```python
from build123d import *

# Parameters (mm, degrees)
F1_DEPTH = 2.7
F3_DEPTH = 6.2
F4_R     = 1.25
F5_DEPTH = 25
F6_SIZE  = 0.5


with BuildPart() as f1:
    # F0 (on Top) → F1 (new body)
    with BuildSketch(Plane.XY):
        with BuildLine():
            Line((-35, -6), (35, -6))
            ThreePointArc((35, -6), (36.3416407865, -5.683281573), (37.4, -4.8))
            ThreePointArc((37.4, -4.8), (39, 0), (37.4, 4.8))
            ThreePointArc((37.4, 4.8), (36.3416407865, 5.683281573), (35, 6))
            Line((35, 6), (-35, 6))
            ThreePointArc((-35, 6), (-36.3416407865, 5.683281573), (-37.4, 4.8))
            ThreePointArc((-37.4, 4.8), (-39, 0), (-37.4, -4.8))
            ThreePointArc((-37.4, -4.8), (-36.3416407865, -5.683281573), (-35, -6))
        make_face()
    extrude(amount=F1_DEPTH)

    # F2 (on face) → F3 (join)
    with BuildSketch(Plane.XY.offset(2.7)):
        with BuildLine():
            Line((29, 4.5), (-29, 4.5))
            ThreePointArc((-29, 4.5), (-31.8284271247, 3.3284271247), (-33, 0.5))
            Line((-33, 0.5), (-33, -0.5))
            ThreePointArc((-33, -0.5), (-31.8284271247, -3.3284271247), (-29, -4.5))
            Line((-29, -4.5), (29, -4.5))
            ThreePointArc((29, -4.5), (31.8284271247, -3.3284271247), (33, -0.5))
            Line((33, -0.5), (33, 0.5))
            ThreePointArc((33, 0.5), (31.8284271247, 3.3284271247), (29, 4.5))
        make_face()
    extrude(amount=F3_DEPTH)

    # F4 (on face) → F5 (cut)
    with BuildSketch(Plane.XY.offset(2.7)):
        with Locations((-36.5, 0)):
            Circle(F4_R)
        with Locations((36.5, 0)):
            Circle(F4_R)
    extrude(amount=-F5_DEPTH, mode=Mode.SUBTRACT)

    # F6
    f6_edges = [f1.edges().sort_by_distance(p)[0] for p in [
        (-37.75, 0, 0),
        (35.25, 0, 0),
    ]]
    chamfer(f6_edges, length=F6_SIZE)


solid = f1.part
```
CAD build for the part. Positions are in the model's coordinates, mm. A direction names the side the tool comes from. Round coordinates to 2 decimals unless told otherwise and drop trailing zeros. Loops run counter-clockwise (first coordinate to the right, second up) from the corner with the lowest first, then second, coordinate; pieces in that order, holes last. Notation, with made-up numbers: M 86,17.25 L 100,17.25 A20 ccw 100,32.25 Z; hole C 89.5,34.5 d5. An arc over 180 degrees is marked long. Use a Markdown table: item, result. Add a question column.
(1) Which spindle directions (+Z, -Z, +X, -X, +Y, -Y) get a long thin tool onto all of the face, cutting with end or side? Do faces 4 (the face through (-31.859, -3.297, 5.757)), 5 (the face through (31.797, -3.359, 5.757)), 6 (the face through (0, -4.5, 6)). Say none if no direction does.
(2) Cut at A-A (z = 1.5). Give the cut face in (x, y), and give its area (3 significant figures).
(3) Cut at D-D (z = 7). Give the cut face in (x, y), and give its area (3 significant figures).
(4) Cut at B-B (x = 10.5). Give the cut face in (y, z).
(5) Pull direction Y, two halves, no side cores. Call faces 1 (the face through (-1, 0, 0)), 2 (the face through (-37.75, 0.05, 1.62)), 3 (the face through (0, -6, 1)): +Y half, -Y half, draft (parallel to the pull), parting line (faces both ways), or undercut.
(6) Drill centre lines: line 1 (Z direction, x = 16.5, y = -5); line 2 (Y direction, x = -25, z = 7.5); line 3 (Y direction, x = 36.5, z = 1.5). Where is each one in solid material? Low to high.
(7) Cut at C-C (x = 36.5). Give the cut face in (y, z), and give its area (3 significant figures).
(8) Flat gauge pins, fed straight in: pin 1 (1.5 mm diameter, centred on y = -2, z = 5, fed in from +X); pin 2 (2 mm diameter, centred on y = 2, z = 4.5, fed in from +X); pin 3 (2 mm diameter, centred on x = 36.5, y = 0, fed in from +Z); pin 4 (1.5 mm diameter, centred on x = 22.5, z = 6.5, fed in from -Y). Where does each tip first touch, or does it go through?
Geometry says:
| question | item | result |
|---|---|---|
| 1 | face 4 | +Z, -X, -Y |
| 1 | face 5 | +Z, +X, -Y |
| 1 | face 6 | +Z, +X, -X, -Y |
| 2 | outline | M -37.4,-4.8 A3 ccw -35,-6 L 35,-6 A3 ccw 37.4,-4.8 A8 ccw 37.4,4.8 A3 ccw 35,6 L -35,6 A3 ccw -37.4,4.8 A8 ccw Z; hole C -36.5,0 d2.5; hole C 36.5,0 d2.5 |
| 2 | area | 905 mm² |
| 3 | outline | M -33,-0.5 A4 ccw -29,-4.5 L 29,-4.5 A4 ccw 33,-0.5 L 33,0.5 A4 ccw 29,4.5 L -29,4.5 A4 ccw -33,0.5 Z |
| 3 | area | 580 mm² |
| 4 | outline | M -6,0 L 6,0 L 6,2.7 L 4.5,2.7 L 4.5,8.9 L -4.5,8.9 L -4.5,2.7 L -6,2.7 Z |
| 5 | face 1 | draft |
| 5 | face 2 | undercut |
| 5 | face 3 | -Y half |
| 6 | line 1 | z = 0 to 2.7 |
| 6 | line 2 | y = -4.5 to 4.5 |
| 6 | line 3 | y = -5.6 to -1.25, 1.25 to 5.6 |
| 7 | outline | M -5.6,0 L -1.75,0 L -1.25,0.5 L -1.25,2.7 L -5.6,2.7 Z; M 1.25,0.5 L 1.75,0 L 5.6,0 L 5.6,2.7 L 1.25,2.7 Z |
| 7 | area | 23.2 mm² |
| 8 | pin 1 | stops at x = 32.93 |
| 8 | pin 2 | stops at x = 32.97 |
| 8 | pin 3 | passes through |
| 8 | pin 4 | stops at y = -4.5 |
